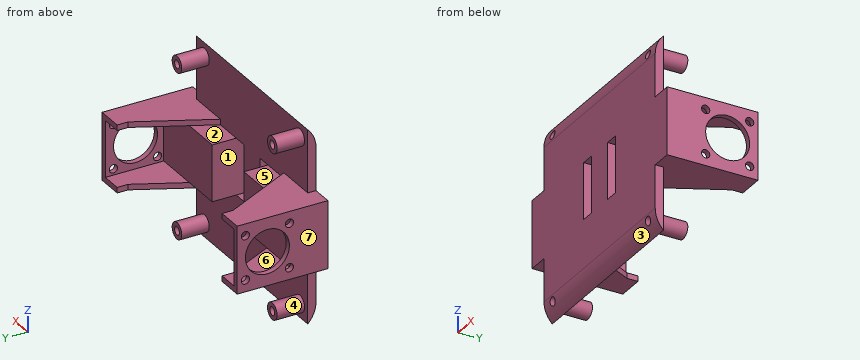
from build123d import *

# Parameters (mm, degrees)
SKETCH1_W                       = 70
SKETCH1_H                       = 70
BOSS_EXTRUDE1_DEPTH             = 3
SKETCH2_W                       = 7.5
SKETCH2_H                       = 20.5
BOSS_EXTRUDE2_DEPTH             = 3
SKETCH3_W                       = 2
SKETCH3_H                       = 20.5
BOSS_EXTRUDE3_DEPTH             = 30
CUT_EXTRUDE1_DEPTH              = 114.481275989
CUT_EXTRUDE1_DEPTH_BACK         = 114.481275989
SKETCH4_R                       = 8
SKETCH4_R_2                     = 1.5
BOSS_EXTRUDE4_REACH             = 110.657
SKETCH5_W                       = 9.5
SKETCH5_H                       = 2
BOSS_EXTRUDE4_DIRECTION_2_REACH = 110.657
BOSS_EXTRUDE5_REACH             = 98.581
SKETCH7_W                       = 81
SKETCH7_H                       = 20.5
CUT_EXTRUDE2_DEPTH              = 109.656569061
SKETCH8_W                       = 5
SKETCH8_H                       = 20.5
CUT_EXTRUDE3_DEPTH              = 109.656569061
BOSS_EXTRUDE7_REACH             = 115.481
SKETCH17_W                      = 20.5
SKETCH17_H                      = 8.75
BOSS_EXTRUDE8_DEPTH             = 30.5
SKETCH19_R                      = 3
BOSS_EXTRUDE9_DEPTH             = 10
SKETCH20_R                      = 1.5
CUT_EXTRUDE4_DEPTH              = 107.330851591
FILLET1_DEPTH                   = 70


with BuildPart() as part:
    # Sketch1 → Boss-Extrude1 (new body)
    with BuildSketch(Plane(origin=(0, 0, 0), x_dir=(1, 0, 0), z_dir=(0, 1, 0))):
        with Locations((35, 35)):
            Rectangle(SKETCH1_W, SKETCH1_H)
    extrude(amount=BOSS_EXTRUDE1_DEPTH)

    # Sketch2 → Boss-Extrude2 (add)
    with BuildSketch(Plane(origin=(0, 3, 0), x_dir=(1, 0, 0), z_dir=(0, 1, 0))):
        with Locations((-3.75, 35)):
            Rectangle(SKETCH2_W, SKETCH2_H)
        with Locations((73.75, 35)):
            Rectangle(SKETCH2_W, SKETCH2_H)
    extrude(amount=-BOSS_EXTRUDE2_DEPTH)

    # Sketch3 → Boss-Extrude3 (add)
    with BuildSketch(Plane(origin=(0, 3, 0), x_dir=(1, 0, 0), z_dir=(0, 1, 0))):
        with Locations((-6.5, 35)):
            Rectangle(SKETCH3_W, SKETCH3_H)
        with Locations((76.5, 35)):
            Rectangle(SKETCH3_W, SKETCH3_H)
    extrude(amount=BOSS_EXTRUDE3_DEPTH)

    # Sketch4 → Cut-Extrude1 (cut, two sides: drawn at the far end of the back side and taken through both)
    with BuildSketch(Plane(origin=(-5.5, 0, 0), x_dir=(0, 0, -1), z_dir=(1, 0, 0)).offset(-CUT_EXTRUDE1_DEPTH_BACK)):
        with Locations((35, 22)):
            Circle(SKETCH4_R)
        with Locations((43, 30)):
            Circle(SKETCH4_R_2)
        with Locations((43, 14)):
            Circle(SKETCH4_R_2)
        with Locations((27, 30)):
            Circle(SKETCH4_R_2)
        with Locations((27, 14)):
            Circle(SKETCH4_R_2)
    extrude(amount=CUT_EXTRUDE1_DEPTH + CUT_EXTRUDE1_DEPTH_BACK, mode=Mode.SUBTRACT)

    # Boss-Extrude4: up to this face of the body (flat: up to its plane)
    boss_extrude4_end = Plane(part.part.faces().sort_by_distance((35, 0, -35))[0])
    # Sketch5 → Boss-Extrude4 (add, up to the picked face)
    with BuildSketch(Plane(origin=(0, 3, 0), x_dir=(1, 0, 0), z_dir=(0, 1, 0)), mode=Mode.PRIVATE) as boss_extrude4_sk1:
        with Locations((-2.75, 23.75)):
            Rectangle(SKETCH5_W, SKETCH5_H)
    boss_extrude4_tool1 = split(extrude(boss_extrude4_sk1.sketch, amount=-BOSS_EXTRUDE4_REACH, mode=Mode.PRIVATE), bisect_by=boss_extrude4_end, keep=Keep.BOTH, mode=Mode.PRIVATE)
    # Sketch5 → Boss-Extrude4 (add, up to the picked face)
    with BuildSketch(Plane(origin=(0, 3, 0), x_dir=(1, 0, 0), z_dir=(0, 1, 0)), mode=Mode.PRIVATE) as boss_extrude4_sk2:
        with Locations((-2.75, 46.25)):
            Rectangle(SKETCH5_W, SKETCH5_H)
    boss_extrude4_tool2 = split(extrude(boss_extrude4_sk2.sketch, amount=-BOSS_EXTRUDE4_REACH, mode=Mode.PRIVATE), bisect_by=boss_extrude4_end, keep=Keep.BOTH, mode=Mode.PRIVATE)
    # Sketch5 → Boss-Extrude4 (add, up to the picked face)
    with BuildSketch(Plane(origin=(0, 3, 0), x_dir=(1, 0, 0), z_dir=(0, 1, 0)), mode=Mode.PRIVATE) as boss_extrude4_sk3:
        with Locations((72.75, 23.75)):
            Rectangle(SKETCH5_W, SKETCH5_H)
    boss_extrude4_tool3 = split(extrude(boss_extrude4_sk3.sketch, amount=-BOSS_EXTRUDE4_REACH, mode=Mode.PRIVATE), bisect_by=boss_extrude4_end, keep=Keep.BOTH, mode=Mode.PRIVATE)
    # Sketch5 → Boss-Extrude4 (add, up to the picked face)
    with BuildSketch(Plane(origin=(0, 3, 0), x_dir=(1, 0, 0), z_dir=(0, 1, 0)), mode=Mode.PRIVATE) as boss_extrude4_sk4:
        with Locations((72.75, 46.25)):
            Rectangle(SKETCH5_W, SKETCH5_H)
    boss_extrude4_tool4 = split(extrude(boss_extrude4_sk4.sketch, amount=-BOSS_EXTRUDE4_REACH, mode=Mode.PRIVATE), bisect_by=boss_extrude4_end, keep=Keep.BOTH, mode=Mode.PRIVATE)
    add(boss_extrude4_tool1.solids().sort_by(Axis((-2.75, 3, -23.75), (0, -1, 0)))[0])
    add(boss_extrude4_tool2.solids().sort_by(Axis((-2.75, 3, -46.25), (0, -1, 0)))[0])
    add(boss_extrude4_tool3.solids().sort_by(Axis((72.75, 3, -23.75), (0, -1, 0)))[0])
    add(boss_extrude4_tool4.solids().sort_by(Axis((72.75, 3, -46.25), (0, -1, 0)))[0])

    # Boss-Extrude4 direction 2: up to this face of the body (flat: up to its plane)
    boss_extrude4_direction_2_end = Plane(part.part.faces().sort_by_distance((76.5, 33, -35))[0])
    # Sketch5 → Boss-Extrude4 direction 2 (add, up to the picked face)
    with BuildSketch(Plane(origin=(0, 3, 0), x_dir=(1, 0, 0), z_dir=(0, 1, 0)), mode=Mode.PRIVATE) as boss_extrude4_direction_2_sk1:
        with Locations((-2.75, 23.75)):
            Rectangle(SKETCH5_W, SKETCH5_H)
    boss_extrude4_direction_2_tool1 = split(extrude(boss_extrude4_direction_2_sk1.sketch, amount=BOSS_EXTRUDE4_DIRECTION_2_REACH, mode=Mode.PRIVATE), bisect_by=boss_extrude4_direction_2_end, keep=Keep.BOTH, mode=Mode.PRIVATE)
    # Sketch5 → Boss-Extrude4 direction 2 (add, up to the picked face)
    with BuildSketch(Plane(origin=(0, 3, 0), x_dir=(1, 0, 0), z_dir=(0, 1, 0)), mode=Mode.PRIVATE) as boss_extrude4_direction_2_sk2:
        with Locations((-2.75, 46.25)):
            Rectangle(SKETCH5_W, SKETCH5_H)
    boss_extrude4_direction_2_tool2 = split(extrude(boss_extrude4_direction_2_sk2.sketch, amount=BOSS_EXTRUDE4_DIRECTION_2_REACH, mode=Mode.PRIVATE), bisect_by=boss_extrude4_direction_2_end, keep=Keep.BOTH, mode=Mode.PRIVATE)
    # Sketch5 → Boss-Extrude4 direction 2 (add, up to the picked face)
    with BuildSketch(Plane(origin=(0, 3, 0), x_dir=(1, 0, 0), z_dir=(0, 1, 0)), mode=Mode.PRIVATE) as boss_extrude4_direction_2_sk3:
        with Locations((72.75, 23.75)):
            Rectangle(SKETCH5_W, SKETCH5_H)
    boss_extrude4_direction_2_tool3 = split(extrude(boss_extrude4_direction_2_sk3.sketch, amount=BOSS_EXTRUDE4_DIRECTION_2_REACH, mode=Mode.PRIVATE), bisect_by=boss_extrude4_direction_2_end, keep=Keep.BOTH, mode=Mode.PRIVATE)
    # Sketch5 → Boss-Extrude4 direction 2 (add, up to the picked face)
    with BuildSketch(Plane(origin=(0, 3, 0), x_dir=(1, 0, 0), z_dir=(0, 1, 0)), mode=Mode.PRIVATE) as boss_extrude4_direction_2_sk4:
        with Locations((72.75, 46.25)):
            Rectangle(SKETCH5_W, SKETCH5_H)
    boss_extrude4_direction_2_tool4 = split(extrude(boss_extrude4_direction_2_sk4.sketch, amount=BOSS_EXTRUDE4_DIRECTION_2_REACH, mode=Mode.PRIVATE), bisect_by=boss_extrude4_direction_2_end, keep=Keep.BOTH, mode=Mode.PRIVATE)
    add(boss_extrude4_direction_2_tool1.solids().sort_by(Axis((-2.75, 3, -23.75), (0, 1, 0)))[0])
    add(boss_extrude4_direction_2_tool2.solids().sort_by(Axis((-2.75, 3, -46.25), (0, 1, 0)))[0])
    add(boss_extrude4_direction_2_tool3.solids().sort_by(Axis((72.75, 3, -23.75), (0, 1, 0)))[0])
    add(boss_extrude4_direction_2_tool4.solids().sort_by(Axis((72.75, 3, -46.25), (0, 1, 0)))[0])

    # Boss-Extrude5: up to this face of the body (flat: up to its plane)
    boss_extrude5_end = Plane(part.part.faces().sort_by_distance((72.823170732, 16.792682927, -22.75))[0])
    # Sketch6 → Boss-Extrude5 (add, up to the picked face)
    with BuildSketch(Plane(origin=(0, 0, -47.25), x_dir=(-1, 0, 0), z_dir=(0, 0, -1)), mode=Mode.PRIVATE) as boss_extrude5_sk1:
        Polygon((-70, 33), (-55, 3), (-70, 3), align=None)
    boss_extrude5_tool1 = split(extrude(boss_extrude5_sk1.sketch, amount=-BOSS_EXTRUDE5_REACH, mode=Mode.PRIVATE), bisect_by=boss_extrude5_end, keep=Keep.BOTH, mode=Mode.PRIVATE)
    # Sketch6 → Boss-Extrude5 (add, up to the picked face)
    with BuildSketch(Plane(origin=(0, 0, -47.25), x_dir=(-1, 0, 0), z_dir=(0, 0, -1)), mode=Mode.PRIVATE) as boss_extrude5_sk2:
        Polygon((0, 33), (-15, 3), (0, 3), align=None)
    boss_extrude5_tool2 = split(extrude(boss_extrude5_sk2.sketch, amount=-BOSS_EXTRUDE5_REACH, mode=Mode.PRIVATE), bisect_by=boss_extrude5_end, keep=Keep.BOTH, mode=Mode.PRIVATE)
    add(boss_extrude5_tool1.solids().sort_by(Axis((65, 13, -47.25), (0, 0, 1)))[0])
    add(boss_extrude5_tool2.solids().sort_by(Axis((5, 13, -47.25), (0, 0, 1)))[0])

    # Sketch7 → Cut-Extrude2 (cut, through all)
    with BuildSketch(Plane(origin=(0, 3, 0), x_dir=(1, 0, 0), z_dir=(0, 1, 0))):
        with Locations((35, 35)):
            Rectangle(SKETCH7_W, SKETCH7_H)
    extrude(amount=CUT_EXTRUDE2_DEPTH, mode=Mode.SUBTRACT)

    # Sketch8 → Cut-Extrude3 (cut, through all)
    with BuildSketch(Plane(origin=(0, 3, 0), x_dir=(1, 0, 0), z_dir=(0, 1, 0))):
        with Locations((27.5, 35)):
            Rectangle(SKETCH8_W, SKETCH8_H)
        with Locations((42.5, 35)):
            Rectangle(SKETCH8_W, SKETCH8_H)
    extrude(amount=-CUT_EXTRUDE3_DEPTH, mode=Mode.SUBTRACT)

    # Boss-Extrude7: up to this face of the body (flat: up to its plane)
    boss_extrude7_end = Plane(part.part.faces().sort_by_distance((45, 1.5, -35))[0])
    # Sketch17 → Boss-Extrude7 (add, up to the picked face)
    with BuildSketch(Plane.ZY.offset(-75.5), mode=Mode.PRIVATE) as boss_extrude7_sk1:
        with Locations((-35, 7.375)):
            Rectangle(SKETCH17_W, SKETCH17_H)
    boss_extrude7_tool1 = split(extrude(boss_extrude7_sk1.sketch, amount=BOSS_EXTRUDE7_REACH, mode=Mode.PRIVATE), bisect_by=boss_extrude7_end, keep=Keep.BOTH, mode=Mode.PRIVATE)
    add(boss_extrude7_tool1.solids().sort_by(Axis((75.5, 7.375, -35), (-1, 0, 0)))[0])

    # Sketch18 → Boss-Extrude8 (add)
    with BuildSketch(Plane(origin=(-5.5, 0, 0), x_dir=(0, 0, -1), z_dir=(1, 0, 0))):
        Polygon((24.75, 3), (24.75, 0), (45.25, 0), (45.25, 3), (45.25, 11.75), (24.75, 11.75), align=None)
    extrude(amount=BOSS_EXTRUDE8_DEPTH)

    # Sketch19 → Boss-Extrude9 (add)
    with BuildSketch(Plane(origin=(0, 3, 0), x_dir=(1, 0, 0), z_dir=(0, 1, 0))):
        with Locations(Location((5, 5, 0), (0, 0, 90))):
            Circle(SKETCH19_R)
        with Locations(Location((65, 5, 0), (0, 0, 90))):
            Circle(SKETCH19_R)
        with Locations(Location((65, 65, 0), (0, 0, 90))):
            Circle(SKETCH19_R)
        with Locations(Location((5, 65, 0), (0, 0, 90))):
            Circle(SKETCH19_R)
    extrude(amount=BOSS_EXTRUDE9_DEPTH)

    # Sketch20 → Cut-Extrude4 (cut, through all)
    with BuildSketch(Plane(origin=(0, 13, 0), x_dir=(1, 0, 0), z_dir=(0, 1, 0))):
        with Locations(Location((5, 65, 0), (0, 0, 270))):
            Circle(SKETCH20_R)
        with Locations(Location((65, 65, 0), (0, 0, 270))):
            Circle(SKETCH20_R)
        with Locations(Location((65, 5, 0), (0, 0, 270))):
            Circle(SKETCH20_R)
        with Locations(Location((5, 5, 0), (0, 0, 270))):
            Circle(SKETCH20_R)
    extrude(amount=-CUT_EXTRUDE4_DEPTH, mode=Mode.SUBTRACT)

    # Fillet1: read off the stored shape, not the designer's step
    # Fillet1 outline → Fillet1 (cut)
    with BuildSketch(Plane.YZ):
        with BuildLine():
            Line((0, 0), (0, -7.141428429))
            ThreePointArc((0, -7.141428429), (0.780455543, -3.268445083), (3, 0))
            Line((3, 0), (0, 0))
        make_face()
        with BuildLine():
            ThreePointArc((3, -70), (0.780455543, -66.731554917), (0, -62.858571571))
            Line((0, -62.858571571), (0, -70))
            Line((0, -70), (3, -70))
        make_face()
    extrude(amount=FILLET1_DEPTH, mode=Mode.SUBTRACT)


solid = part.part
For this review, take the finished solid that the model builds, in its own axes (mm). Face numbers are marked on the shaded views. A direction names the side the tool comes from. Give positions to 0.01 mm unless a question says otherwise; leave off trailing zeros. Order: outer loops, then holes, each group sorted by start corner. A loop starts at its lowest first (then second) coordinate and runs counter-clockwise, first axis right, second up. Notation, with made-up numbers: (-16, 62) -> (20, 62) arc R30 cw to (20, 91) -> close; hole circle Ø9 at (77, 39). An arc over 180 degrees is marked (long way). Write item = value, one per line.
1) We need section A-A, the plane y = 22. Give the boundary of the cut face in (x, z).
Findings:
outline = (-7.5, -47.25) -> (5.5, -47.25) -> (5.5, -45.25) -> (-5.5, -45.25) -> (-5.5, -43) -> (-7.5, -43) -> close; (-7.5, -27) -> (-5.5, -27) -> (-5.5, -24.75) -> (5.5, -24.75) -> (5.5, -22.75) -> (-7.5, -22.75) -> close; (64.5, -47.25) -> (77.5, -47.25) -> (77.5, -43) -> (75.5, -43) -> (75.5, -45.25) -> (64.5, -45.25) -> close; (64.5, -24.75) -> (75.5, -24.75) -> (75.5, -27) -> (77.5, -27) -> (77.5, -22.75) -> (64.5, -22.75) -> close
2) We need section D-D, the plane x = 5. Give the boundary of the cut face in (y, z).
Findings:
outline = (0, -62.86) arc R10 ccw to (0.02, -63.5) -> (13, -63.5) -> (13, -62) -> (3, -62) -> (3, -47.25) -> (23, -47.25) -> (23, -45.25) -> (11.75, -45.25) -> (11.75, -24.75) -> (23, -24.75) -> (23, -22.75) -> (3, -22.75) -> (3, -8) -> (13, -8) -> (13, -6.5) -> (0.02, -6.5) arc R10 ccw to (0, -7.14) -> close; (0.69, -66.5) arc R10 ccw to (3, -70) -> (3, -68) -> (13, -68) -> (13, -66.5) -> close; (0.69, -3.5) -> (13, -3.5) -> (13, -2) -> (3, -2) -> (3, 0) arc R10 ccw to start
3) We need section C-C, the plane z = -65. Give the boundary of the cut face in (x, y), and give its area (3 significant figures).
Findings:
outline = (0, 0.23) -> (3.5, 0.23) -> (3.5, 13) -> (2, 13) -> (2, 3) -> (0, 3) -> close; (6.5, 0.23) -> (63.5, 0.23) -> (63.5, 13) -> (62, 13) -> (62, 3) -> (8, 3) -> (8, 13) -> (6.5, 13) -> close; (66.5, 0.23) -> (70, 0.23) -> (70, 3) -> (68, 3) -> (68, 13) -> (66.5, 13) -> close
area = 237 mm^2
4) For the marked faces 1, 2, 3 and 4, list the 3-axis set-ups (+Z, -Z, +X, -X, +Y, -Y) from which the entire face can be reached by the end or side of a thin tool; tool diameter is ignored.
Findings:
face_1 = +Y, -Y
face_2 = +Z, +Y
face_3 = -Z, +X, -X, -Y
face_4 = +Y
5) To check wall thickness, follow L1, parallel to Z at x = 65, y = 3.5; L2, parallel to X at y = 5.75, z = -5; L3, parallel to Z at x = 73, y = 15. State the ranges of each line that lie inside material, in increasing order. Write a range as from..to.
Findings:
L1 = -68..-66.5, -63.5..-62, -47.25..-22.75, -8..-6.5, -3.5..-2
L2 = 2..3.5, 6.5..8, 62..63.5, 66.5..68
L3 = -47.25..-45.25, -24.75..-22.75
6) Insertion check: pin 1 (2 mm diameter, centred on x = 9.5, z = -52.5, fed in from +Y); pin 2 (6.5 mm diameter, centred on x = 6, z = -4, fed in from +Y); pin 3 (2.5 mm diameter, centred on x = 14.5, y = 7.5, fed in from -Z); pin 4 (6 mm diameter, centred on y = 27.5, z = -37.5, fed in from +X). Each pin has a flat end and moves straight along its axis. Give the tip position at first contact, or say it passes through.
Findings:
pin_1 = 3
pin_2 = 13
pin_3 = -45.25
pin_4 = 77.5
7) Draft analysis for pull direction Z (two halves, no side actions). For the marked faces 5, 6 and 7, state which applies: pulls with the +Z half, pulls with the -Z half, needs draft (parallel to the pull), parting line crosses it, or undercut.
Findings:
face_5 = pulls with the +Z half
face_6 = undercut
face_7 = needs draft
8) We need section B-B, the plane x = 47. Give the boundary of the cut face in (y, z), and give its area (3 significant figures).
Findings:
outline = (0, -62.86) arc R10 ccw to (3, -70) -> (3, -45.25) -> (11.75, -45.25) -> (11.75, -24.75) -> (3, -24.75) -> (3, 0) arc R10 ccw to (0, -7.14) -> close
area = 376 mm^2
